```python
from build123d import *

# Parameters (mm, degrees)
EXTRUDE_1_DEPTH     = 20
EXTRUDE_2_DEPTH     = 3.5
CUT_EXTRUDE_2_DEPTH = 35.234485537
CUT_EXTRUDE_3_DEPTH = 35.234485537


with BuildPart() as part:
    # 草图1 → 凸台-拉伸1 (new body)
    with BuildSketch(Plane.XY):
        Polygon((14, -14), (-14, -14), (-14, -10), (10, -10), (10, 14), (14, 14), align=None)
    extrude(amount=EXTRUDE_1_DEPTH)

    # 草图3 → 凸台-拉伸2 (add)
    with BuildSketch(Plane(origin=(0, 0, 0), x_dir=(-1, 0, 0), z_dir=(0, 0, -1))):
        Polygon((-10, 14), (-7.7, 14), (-7.7, 9.5), (9.5, -7.7), (14, -7.7), (14, -10), (14, -14), (-14, -14), (-14, 14), align=None)
    extrude_2 = extrude(amount=-EXTRUDE_2_DEPTH)

    # 镜向2: 凸台-拉伸2 across plane
    add(extrude_2.mirror(Plane.XY.offset(10)))

    # 草图6 → 切除-拉伸2 (cut, through all)
    with BuildSketch(Plane.ZY.offset(-10)):
        with BuildLine():
            Line((13.25, 4), (13.25, -1))
            ThreePointArc((13.25, -1), (10, -4.25), (6.75, -1))
            Line((6.75, -1), (6.75, 4))
            ThreePointArc((6.75, 4), (10, 7.25), (13.25, 4))
        make_face()
    extrude(amount=-CUT_EXTRUDE_2_DEPTH, mode=Mode.SUBTRACT)

    # 草图8 → 切除-拉伸3 (cut, through all)
    with BuildSketch(Plane(origin=(0, -10, 0), x_dir=(1, 0, 0), z_dir=(0, 1, 0))):
        with BuildLine():
            Line((-4, -6.75), (1, -6.75))
            ThreePointArc((1, -6.75), (4.25, -10), (1, -13.25))
            Line((1, -13.25), (-4, -13.25))
            ThreePointArc((-4, -13.25), (-7.25, -10), (-4, -6.75))
        make_face()
    extrude(amount=-CUT_EXTRUDE_3_DEPTH, mode=Mode.SUBTRACT)


solid = part.part
```
Geometry check sheet. Reference: the model listing, model coordinates, mm. A direction names the side the tool comes from. Round coordinates to 2 decimals unless told otherwise and drop trailing zeros. Order: outer loops, then holes, each group sorted by start corner. A loop starts at its lowest first (then second) coordinate and runs counter-clockwise, first axis right, second up. Notation, with made-up numbers: M 60.5,-7.5 L 75.5,-7.5 A12 cw 75.5,8.5 Z; hole C 82.5,52 d6. An arc over 180 degrees is marked long. Write item = value, one per line.
Q1. Set-up check for faces 4 (the flat face through (3, -3, 3.5)), 5 (the flat face through (12, 1, 6.75)), 6 (the flat face through (7.7, 12, 2)), 7 (the cylindrical face through (-7.25, -11.97, 10.07)): record each of +Z, -Z, +X, -X, +Y, -Y from which the full face is reachable in a straight line by a thin tool's end or side.
Answer block:
face_4 = -X, +Y
face_5 = +X, -X
face_6 = +Z, -Z, -X, +Y
face_7 = +Y, -Y
Q2. Section check A-A (z = 10). Enter the section's corners in (x, y).
Answer block:
outline = M -14,-14 L -7.25,-14 L -7.25,-10 L -14,-10 Z; M 4.25,-14 L 14,-14 L 14,-4.25 L 10,-4.25 L 10,-10 L 4.25,-10 Z; M 10,7.25 L 14,7.25 L 14,14 L 10,14 Z
Q3. Depth check by flat-ended pin: pin 1 Ø4 at (x, z) = (-4.5, 7) entering from +Y; pin 2 Ø3 at (y, z) = (12.5, 18) entering from -X; pin 3 Ø3 at (x, z) = (-11.5, 2.5) entering from +Y. Enter the tip coordinate at first touch or a pass-through.
Answer block:
pin_1 = -10
pin_2 = 7.7
pin_3 = -7.7
Q4. Section check D-D (y = 8.75). Enter the section's corners in (x, z).
Answer block:
outline = M 6.95,0 L 14,0 L 14,20 L 6.95,20 L 6.95,16.5 L 10,16.5 L 10,3.5 L 6.95,3.5 Z
Q5. Section check B-B (y = 0). Enter the section's corners in (x, z), plus the area to 3 significant figures.
Answer block:
outline = M -1.8,0 L 14,0 L 14,6.75 L 10,6.75 L 10,3.5 L -1.8,3.5 Z; M -1.8,16.5 L 10,16.5 L 10,13.25 L 14,13.25 L 14,20 L -1.8,20 Z
area = 137 mm^2
Q6. Section check C-C (x = 9.5). Enter the section's corners in (y, z).
Answer block:
outline = M -14,0 L 14,0 L 14,3.5 L -10,3.5 L -10,16.5 L 14,16.5 L 14,20 L -14,20 Z
Q7. Release check for a two-part mould opening along Z. For faces 1 (the flat face through (-12, -7.7, 2)), 2 (the flat face through (-2, -10, 6)), 3 (the flat face through (3, -3, 0)) record: released by +Z, released by -Z, zero draft, split by the parting line, or undercut.
Answer block:
face_1 = zero draft
face_2 = undercut
face_3 = released by -Z
Q8. Scan lines: line 1 (Z direction, x = 4.5, y = 3); line 2 (Z direction, x = 10.5, y = 0); line 3 (Y direction, x = -7.5, z = 5.25). Record each from-to range of solid material in increasing order.
Answer block:
line_1 = 0 to 3.5, 16.5 to 20
line_2 = 0 to 6.75, 13.25 to 20
line_3 = -14 to -10
